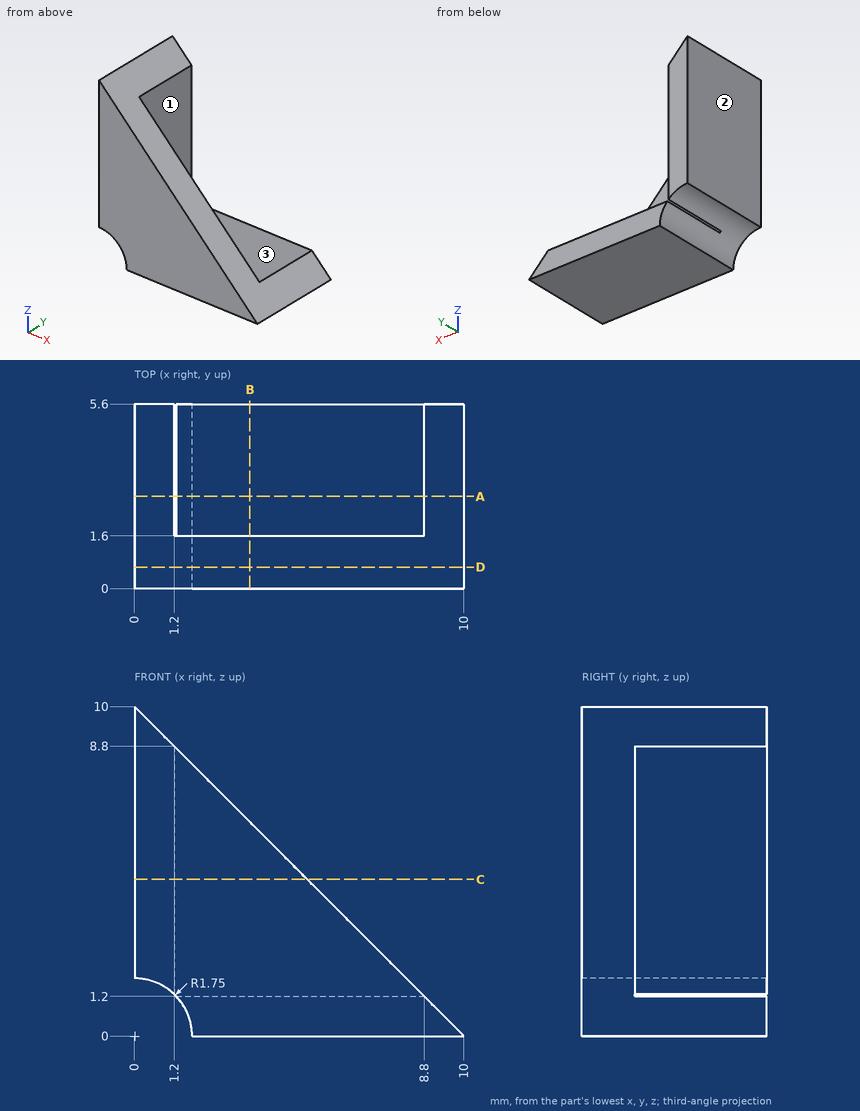
Print and shaded views of the part. All mm, measured from the part's lowest x, y and z. A direction names the side the tool comes from. Give positions to 0.01 mm unless a question says otherwise; leave off trailing zeros. Write each loop counter-clockwise with the first axis right and the second up, starting at its lowest first coordinate (ties: lowest second). Pieces come first, ordered by that corner, then holes. Notation, with made-up numbers: (79.25, 53.25) - (115.25, 53.25) arc R13 cw to (115.25, 60.25) - close; hole circle Ø6 at (12, 17). An arc over 180 degrees is marked (long way). One line per question, with ' | ' between items. Start each with the question number.
(1) Wall check: line 1 along X through (y, z) = (3.8, 3.5); line 2 along Y through (x, z) = (7, 1.5). Give the ranges that are in metal, low to high. Write a range as from..to.
(2) Pin check, flat tips, straight feed: P1, Ø1.5, axis at y = 2.5, z = 5, coming from the +X side; P2, Ø1.2, axis at x = 6, y = 3, coming from the +Z side; P3, Ø1, axis at x = 2, y = 3, coming from the -Z side; P4, Ø1.5, axis at x = 6, z = 2, coming from the +Y side. Stop position of each tip, or through.
(3) Slice it at D-D on y = 0.65. Write the cut outline in (x, z).
(4) 3-axis set-ups, long thin cutter, end or side, ignore diameter. For the marked faces 1, 2 and 3: which of +Z, -Z, +X, -X, +Y, -Y reach the whole face in a straight line?
(5) Slice it at C-C on z = 4.75. Write the cut outline in (x, y), plus the area to 3 significant figures.
(6) Slice it at B-B on x = 3.5. Write the cut outline in (y, z), plus the area to 3 significant figures.
(7) Slice it at A-A on y = 2.8. Write the cut outline in (x, z), plus the area to 3 significant figures.
Results below:
1) line 1: 0..1.2 | line 2: 0..1.6
2) P1: x = 1.2 | P2: z = 1.2 | P3: z = 0 | P4: y = 1.6
3) outline: (0, 1.75) arc R1.75 cw to (1.75, 0) - (10, 0) - (0, 10) - close
4) face 1: +Z, -Z, +X, +Y | face 2: +Z, -Z, -X, +Y, -Y | face 3: +Z, +X, -X, +Y
5) outline: (0, 0) - (5.25, 0) - (5.25, 1.6) - (1.2, 1.6) - (1.2, 5.6) - (0, 5.6) - close | area: 13.2 mm^2
6) outline: (0, 0) - (5.6, 0) - (5.6, 1.2) - (1.6, 1.2) - (1.6, 6.5) - (0, 6.5) - close | area: 15.2 mm^2
7) outline: (0, 1.75) arc R1.75 cw to (1.2, 1.27) - (1.2, 8.8) - (0, 10) - close; (1.27, 1.2) arc R1.75 cw to (1.75, 0) - (10, 0) - (8.8, 1.2) - close | area: 18.7 mm^2
